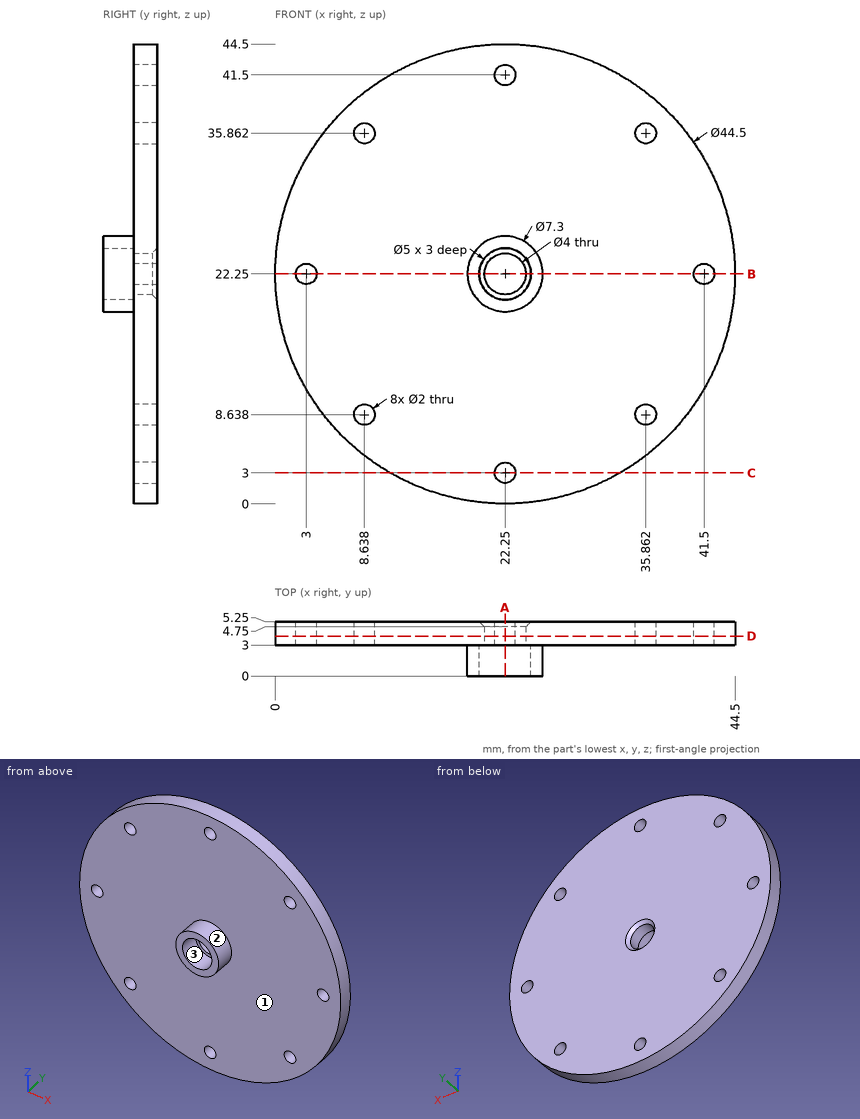
Drawing for the job (mm, zero at the part's lowest x, y, z). Give positions to 0.01 mm unless a question says otherwise; leave off trailing zeros. Write each loop counter-clockwise with the first axis right and the second up, starting at its lowest first coordinate (ties: lowest second). Pieces come first, ordered by that corner, then holes. Notation, with made-up numbers: M -5.75,-3.5 L 48.25,-3.5 A17 ccw 48.25,1.5 Z; hole C 34,70.5 d3. An arc over 180 degrees is marked long. Return JSON: item names as keys, results as strings. Group by question number.
(1) Drill centre lines: L1, parallel to X at y = 4.2, z = 22.25; L2, parallel to X at y = 4.5, z = 9.5 (1 decimal); L3, parallel to X at y = 2.2, z = 22.25. Where is each one in solid material? Low to high. Write a range as [from, to].
(2) Mould opens along Z. For the marked faces 1, 2 and 3 say: pulls with the +Z half, pulls with the -Z half, needs draft (parallel to the pull), parting line crosses it, or undercut.
(3) Band-saw the part on C-C (z = 3). Give the cut face in (x, y).
(4) Band-saw the part on B-B (z = 22.25). Give the cut face in (x, y).
(5) Band-saw the part on D-D (y = 3.85). State how many separate pieces and enclosed holes the cut face has, and give its area (3 significant figures).
(6) Band-saw the part on A-A (x = 22.25). Give the cut face in (y, z).
(7) Flat gauge pins, fed straight in: pin 1 Ø4.5 at (x, z) = (22.25, 22.25) entering from +Y; pin 2 Ø1.6 at (x, z) = (3, 22.25) entering from -Y; pin 3 Ø2.5 at (x, z) = (35.86, 8.64) entering from -Y; pin 4 Ø1.5 at (x, y) = (15, 4) entering from +Z. Where does each tip first touch, or does it go through?
Entries:
{
 "1": {"L1": "x = [0, 2], [4, 20.25], [24.25, 40.5], [42.5, 44.5]", "L2": "x = [4, 8.1], [9.1, 35.4], [36.4, 40.5]", "L3": "x = [18.6, 19.75], [24.75, 25.9]"},
 "2": {"face 1": "needs draft", "face 2": "parting line crosses it", "face 3": "undercut"},
 "3": {"outline": "M 11.09,3 L 21.25,3 L 21.25,5.25 L 11.09,5.25 Z; M 23.25,3 L 33.41,3 L 33.41,5.25 L 23.25,5.25 Z"},
 "4": {"outline": "M 0,3 L 2,3 L 2,5.25 L 0,5.25 Z; M 4,3 L 18.6,3 L 18.6,0 L 19.75,0 L 19.75,3 L 20.25,3 L 20.25,4.75 L 19.75,5.25 L 4,5.25 Z; M 24.25,3 L 24.75,3 L 24.75,0 L 25.9,0 L 25.9,3 L 40.5,3 L 40.5,5.25 L 24.75,5.25 L 24.25,4.75 Z; M 42.5,3 L 44.5,3 L 44.5,5.25 L 42.5,5.25 Z"},
 "5": {"separate pieces": "1", "enclosed holes": "9", "area": "1,520 mm^2"},
 "6": {"outline": "M 0,18.6 L 3,18.6 L 3,4 L 5.25,4 L 5.25,19.75 L 4.75,20.25 L 3,20.25 L 3,19.75 L 0,19.75 Z; M 0,24.75 L 3,24.75 L 3,24.25 L 4.75,24.25 L 5.25,24.75 L 5.25,40.5 L 3,40.5 L 3,25.9 L 0,25.9 Z; M 3,0 L 5.25,0 L 5.25,2 L 3,2 Z; M 3,42.5 L 5.25,42.5 L 5.25,44.5 L 3,44.5 Z"},
 "7": {"pin 1": "stops at y = 5", "pin 2": "passes through", "pin 3": "stops at y = 3", "pin 4": "stops at z = 43.53"}
}
